from build123d import *

# Parameters (mm, degrees)
SKETCH1_R           = 6.35
EXTRUDE1_DEPTH      = 38.1
CHAMFER1_SIZE       = 0.9525
SKETCH3_W           = 3.175
SKETCH3_H           = 1.5875
EXTRUDE2_DEPTH      = 39.1
EXTRUDE2_DEPTH_BACK = 39.1


with BuildPart() as part:
    # Sketch1 → Extrude1 (new body, symmetric)
    with BuildSketch(Plane.XY):
        Circle(SKETCH1_R)
    extrude(amount=EXTRUDE1_DEPTH, both=True)

    # Chamfer1
    chamfer1_edges = [part.edges().sort_by_distance(p)[0] for p in [
        (-6.35, 0, -38.1),
        (-6.35, 0, 38.1),
    ]]
    chamfer(chamfer1_edges, length=CHAMFER1_SIZE)

    # Sketch3 → Extrude2 (cut, two sides)
    with BuildSketch(Plane.XY) as extrude2_sk:
        with Locations((0, 5.55625)):
            Rectangle(SKETCH3_W, SKETCH3_H)
    extrude(amount=EXTRUDE2_DEPTH, mode=Mode.SUBTRACT)
    extrude(extrude2_sk.sketch, amount=-EXTRUDE2_DEPTH_BACK, mode=Mode.SUBTRACT)


solid = part.part
Input: part model. Units: mm. Frame: model coordinates. A direction names the side the tool comes from. Coordinates: 2 decimals unless noted, no trailing zeros. Loops run counter-clockwise (first coordinate to the right, second up) from the corner with the lowest first, then second, coordinate; pieces in that order, holes last. Notation, with made-up numbers: (23, 43) -> (49, 43) arc R25 cw to (49, 61) -> close; hole circle Ø2 at (63.25, -7). An arc over 180 degrees is marked (long way). Write item = value, one per line. Start each with the question number.
Item 1: Cut plane A-A, the plane x = 0. Return loops of the section in (y, z).
Item 2: Mould query, pull axis X, two halves, no side actions, for faces 1 (the face through (0, 0, 38.1)), 2 (the face through (-0.257, -6.345, 0.52)), 3 (the face through (-1.588, 5, 1)), 4 (the face through (0, 4.762, -1)). Classes: pulls with the +X half, pulls with the -X half, needs draft (parallel to the pull), parting line crosses it, or undercut.
Item 3: Material intervals for line 1 (Y direction, x = -1.5, z = 28); line 2 (Z direction, x = 4.5, y = -3.25); line 3 (Y direction, x = 2.5, z = -14.5), sorted ascending.
Item 4: Reachability of faces 5 (the face through (1.588, 5, -1)), 6 (the face through (0, 0, -38.1)) from +Z, -Z, +X, -X, +Y, -Y: full face, straight path, thin tool, end or side. Return the list, or none.
Item 5: First-contact query: P1, Ø1.5, axis at x = 4.5, z = -22.5, coming from the +Y side; P2, Ø2, axis at y = 2, z = -21.5, coming from the -X side; P3, Ø1.1, axis at y = 5, z = 11, coming from the +X side. Flat tips, straight axial feed; report the tip coordinate or a pass-through.
Item 6: Cut plane B-B, the plane z = 20. Return loops of the section in (x, y), plus the area to 3 significant figures.
Ans:
q1.outline = (-6.35, -37.15) -> (-5.4, -38.1) -> (4.76, -38.1) -> (4.76, 38.1) -> (-5.4, 38.1) -> (-6.35, 37.15) -> close
q2.face_1 = needs draft
q2.face_2 = parting line crosses it
q2.face_3 = undercut
q2.face_4 = undercut
q3.line_1 = -6.17 to 4.76
q3.line_2 = -37.95 to 37.95
q3.line_3 = -5.84 to 5.84
q4.face_5 = +Z, -Z, +Y
q4.face_6 = -Z, +X, -X, +Y, -Y
q5.P1 = 5.12
q5.P2 = -6.27
q5.P3 = 4.53
q6.outline = (-1.59, 4.76) -> (-1.59, 6.15) arc R6.35 ccw (long way) to (1.59, 6.15) -> (1.59, 4.76) -> close
q6.area = 122 mm²
